```python
from build123d import *

# Parameters (mm, degrees)
BOSS_EXTRUDE1_DEPTH     = 200
CUT_EXTRUDE1_DEPTH      = 77.2000001
CUT_EXTRUDE1_DEPTH_BACK = 77.2000001


with BuildPart() as part:
    # Sketch17 → Boss-Extrude1 (new body)
    with BuildSketch(Plane.XY):
        with BuildLine():
            Line((-76.2, -15), (76.2, -15))
            Line((76.2, -15), (76.2, -104.498366301))
            add(Edge.make_bspline(
                [(-76.2, -104.498366301), (0, -115.791283906), (76.2, -104.498366301)],
                knots=[1.253188337, 1.253188337, 1.253188337, 1.888404317, 1.888404317, 1.888404317], degree=2, weights=[1, 0.949985148, 1]))
            Line((-76.2, -104.498366301), (-76.2, -15))
        make_face()
    extrude(amount=-BOSS_EXTRUDE1_DEPTH)

    # Sketch15 → Cut-Extrude1 (cut, two sides)
    with BuildSketch(Plane(origin=(0, 0, 0), x_dir=(0, 0, -1), z_dir=(1, 0, 0))) as cut_extrude1_sk:
        Polygon((0, -110), (200, -110), (200, -95), (0, -105), align=None)
    extrude(amount=CUT_EXTRUDE1_DEPTH, mode=Mode.SUBTRACT)
    extrude(cut_extrude1_sk.sketch, amount=-CUT_EXTRUDE1_DEPTH_BACK, mode=Mode.SUBTRACT)


solid = part.part
```
Here's how the part is built. I have some questions about the finished solid (model axes, mm). Give positions to 0.01 mm unless a question says otherwise; leave off trailing zeros. Order: outer loops, then holes, each group sorted by start corner. A loop starts at its lowest first (then second) coordinate and runs counter-clockwise, first axis right, second up. Notation, with made-up numbers: (17, -17) -> (76, -17) arc R16 ccw to (76, 14) -> close; hole circle Ø8 at (30.5, -2.75). An arc over 180 degrees is marked (long way). Use CSV: the item, a comma, the result in double quotes. Start each with the question number.
Item 1: Suppose I cut it at A-A (x = 7). List the corners of the cut face in (y, z) for me, and give its area (3 significant figures).
Item 2: I'm going to push flat-ended pins straight in: P1, Ø1, axis at x = 56, y = -91, coming from the +Z side; P2, Ø3, axis at x = 13.5, z = -77.5, coming from the -Y side. Where does each tip first touch, or does it pass through?
Item 3: Suppose I cut it at B-B (z = -161). List the corners of the cut face in (x, y) for me.
Item 4: If I drill on probe 1 along Y at (x, z) = (69.5, -9.5) (3 decimals); probe 2 along Y at (x, z) = (-41.5, -173), over which ranges is the centre line in solid material (lowest first)? Write a range as [from, to].
Answer block:
1,outline,"(-105, 0) -> (-95, -200) -> (-15, -200) -> (-15, 0) -> close"
1,area,"17,000 mm^2"
2,P1,"stops at z = 0"
2,P2,"stops at y = -101.2"
3,outline,"(-76.2, -96.95) -> (76.2, -96.95) -> (76.2, -15) -> (-76.2, -15) -> close"
4,probe 1,"y = [-104.525, -15]"
4,probe 2,"y = [-96.35, -15]"
